Geometry check sheet. Reference: the model listing, model coordinates, mm. Give positions to 0.01 mm unless a question says otherwise; leave off trailing zeros. Write each loop counter-clockwise with the first axis right and the second up, starting at its lowest first coordinate (ties: lowest second). Pieces come first, ordered by that corner, then holes. Notation, with made-up numbers: M 59,-38.5 L 64,-38.5 A26 cw 64,-23.5 Z; hole C 0,-1 d6. An arc over 180 degrees is marked long. One line per item, written item: value. Start each with the question number.
1. Cross-section at C-C on x = 0. Record the cut outline in (y, z), then the cut area to 3 significant figures.
2. Scan lines: line 1 (Z direction, x = -44.45, y = 1.25); line 2 (X direction, y = 0.7, z = 1); line 3 (Z direction, x = -32, y = 0.8). Record each from-to range of solid material in increasing order.
3. Cross-section at D-D on z = 40. Record the cut outline in (x, y), then the cut area to 3 significant figures.
4. Gauge pin test, flat ends, axial feed: pin 1 (0.8 mm diameter, centred on y = 1, z = -12, fed in from +X); pin 2 (0.5 mm diameter, centred on y = 1, z = 26.5, fed in from +X). Record the tip position at first contact, or that the pin passes through.
5. Cross-section at A-A on y = 1.2. Count the separate pieces of the cut face and the enclosed holes in it, then the cut area to 3 significant figures.
6. Cross-section at B-B on x = -44.45. Record the cut outline in (y, z), then the cut area to 3 significant figures.
Autodesk Inventor part; units mm, degrees
ref_plane "YZ Plane" through (0, 0, 0) normal (1, 0, 0) x (0, 1, 0)
ref_plane "XZ Plane" through (0, 0, 0) normal (0, 1, 0) x (-1, 0, 0)
ref_plane "XY Plane" through (0, 0, 0) normal (0, 0, 1) x (1, 0, 0)
sketch "main" plane through (0, 0, 0) normal (0, 0, 1) x (1, 0, 0)
  arc A0 (21.831, -6.1969) -> (19.4626, -4.8147) centre (20.2435, -6.1969) ccw
  line L0 (4.5808, -13.2233) -> (19.4626, -4.8147)
  circle A1 centre (-16.269, -6.907) radius 2.0955
  arc A2 (-21.7728, -3.7399) -> (-20.3351, -11.7845) centre (-16.269, -6.907) ccw
  line L1 (34.531, -43.9625) -> (34.531, 70.3375)
  arc A3 (-5.5129, -0.9469) -> (-3.356, -3.1208) centre (-4.137, -1.7387) ccw
  line L2 (-3.356, -3.1208) -> (21.0244, 10.6548)
  arc A4 (21.0244, 10.6548) -> (21.831, 12.037) centre (20.2435, 12.037) ccw
  line L3 (21.831, 12.037) -> (21.831, 40.6294)
  line L4 (18.8676, 41.4212) -> (-5.5129, -0.9469)
  line L5 (-21.7728, -3.7399) -> (22.6772, 73.5046)
  arc A5 (21.831, 40.6294) -> (18.8676, 41.4212) centre (20.2435, 40.6294) ccw
  circle A6 centre (28.181, 70.3375) radius 2.0955
  arc A7 (34.531, 70.3375) -> (22.6772, 73.5046) centre (28.181, 70.3375) ccw
  circle A8 centre (28.181, -43.9625) radius 2.1844
  arc A9 (24.1149, -48.84) -> (34.531, -43.9625) centre (28.181, -43.9625) ccw
  line L6 (24.1149, -48.84) -> (-20.3351, -11.7845)
  arc A10 (4.5808, -13.2233) -> (4.3452, -15.8248) centre (5.3617, -14.6055) ccw
  line L7 (21.831, -27.0116) -> (21.831, -6.1969)
  arc A11 (19.227, -28.2309) -> (21.831, -27.0116) centre (20.2435, -27.0116) ccw
  line L8 (4.3452, -15.8248) -> (19.227, -28.2309)
  point P0 (5.1171, -4.3382)
  point P1 (1.8899, -30.3122)
  point P2 (11.7861, -22.0279)
  dimension "d1" = 12.7
  dimension "d2" = 12.7
  dimension "d3" = 12.7
  dimension "d4" = 1.5875
  dimension "d5" = 12.7
  dimension "d6" = 1.5875
  dimension "d7" = 1.5875
  dimension "d10" = 114.3
  dimension "d12" = 12.7
  dimension "d13" = 12.7
  dimension "d14" = 13.187
  dimension "d16" = 44.45
  dimension "d17" = 12.7
sketch "Sketch1" plane through (0, 0, 0) normal (0, 1, 0) x (-1, 0, 0)
  arc A0 (38.1, 0.7102) -> (35.7316, 2.0923) centre (36.5125, 0.7102) ccw
  line L0 (20.8498, -6.3163) -> (35.7316, 2.0923)
  circle A1 centre (0, 0) radius 2.0955
  arc A2 (-5.5038, 3.1671) -> (-4.0661, -4.8775) centre (0, 0) ccw
  line L1 (50.8, -37.0554) -> (50.8, 77.2446)
  arc A3 (10.7561, 5.9602) -> (12.9129, 3.7863) centre (12.132, 5.1684) ccw
  line L2 (12.9129, 3.7863) -> (37.2934, 17.5619)
  arc A4 (37.2934, 17.5619) -> (38.1, 18.944) centre (36.5125, 18.944) ccw
  line L3 (38.1, 18.944) -> (38.1, 47.5364)
  line L4 (35.1366, 48.3282) -> (10.7561, 5.9602)
  line L5 (-5.5038, 3.1671) -> (38.9462, 80.4117)
  arc A5 (38.1, 47.5364) -> (35.1366, 48.3282) centre (36.5125, 47.5364) ccw
  circle A6 centre (44.45, 77.2446) radius 2.0955
  arc A7 (50.8, 77.2446) -> (38.9462, 80.4117) centre (44.45, 77.2446) ccw
  circle A8 centre (44.45, -37.0554) radius 2.1844
  arc A9 (40.3839, -41.9329) -> (50.8, -37.0554) centre (44.45, -37.0554) ccw
  line L6 (40.3839, -41.9329) -> (-4.0661, -4.8775)
  arc A10 (20.8498, -6.3163) -> (20.6142, -8.9178) centre (21.6307, -7.6984) ccw
  line L7 (38.1, -20.1045) -> (38.1, 0.7102)
  arc A11 (35.496, -21.3239) -> (38.1, -20.1045) centre (36.5125, -20.1045) ccw
  line L8 (20.6142, -8.9178) -> (35.496, -21.3239)
extrude "Extrusion1" add sketch "Sketch1" along normal blind 1.5875
properties part number "gusset" material "Acetal Resin, White"
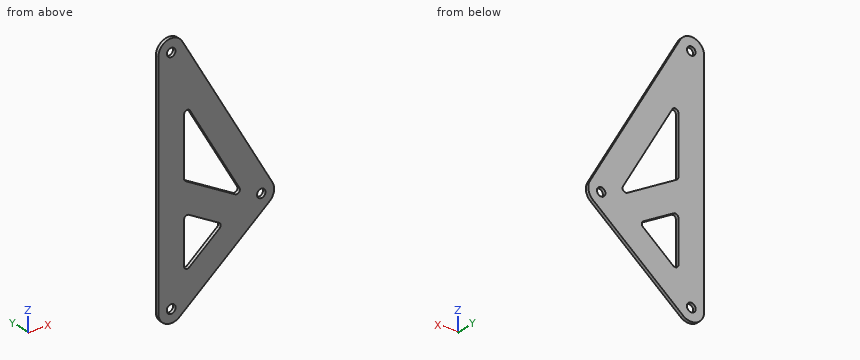
Report:
1. outline: M 0,-8.27 L 1.59,-8.27 L 1.59,-2.1 L 0,-2.1 Z; M 0,2.1 L 1.59,2.1 L 1.59,12.73 L 0,12.73 Z
1. area: 26.7 mm^2
2. line 1: z = -43.41 to -39.24, -34.87 to 75.15, 79.34 to 83.59
2. line 2: x = -50.8 to -38.07, -33.8 to -1.84, 1.84 to 6.27
2. line 3: z = -34.94 to -18.41, -0.02 to 14.57, 42.88 to 68.34
3. outline: M -50.8,0 L -38.1,0 L -38.1,1.59 L -50.8,1.59 Z; M -30.34,0 L -15.69,0 L -15.69,1.59 L -30.34,1.59 Z
3. area: 43.4 mm^2
4. pin 1: stops at x = -4
4. pin 2: stops at x = -7.78
5. separate pieces: 1
5. enclosed holes: 5
5. area: 3,510 mm^2
6. outline: M 0,-43.41 L 1.59,-43.41 L 1.59,-39.24 L 0,-39.24 Z; M 0,-34.87 L 1.59,-34.87 L 1.59,75.15 L 0,75.15 Z; M 0,79.34 L 1.59,79.34 L 1.59,83.59 L 0,83.59 Z
6. area: 188 mm^2
